The model under review builds one solid part; all positions refer to its coordinate system, in mm. A direction names the side the tool comes from. Coordinates: 2 decimals unless noted, no trailing zeros. Write each loop counter-clockwise with the first axis right and the second up, starting at its lowest first coordinate (ties: lowest second). Pieces come first, ordered by that corner, then holes. Notation, with made-up numbers: (69.5, 66) -> (74.5, 66) arc R24 cw to (74.5, 94) -> close; hole circle Ø9 at (56, 89.25). An arc over 180 degrees is marked (long way). Write each question's results on one line, items separated by ' | '.
Autodesk Inventor part; units mm, degrees
ref_plane "YZ Plane" through (0, 0, 0) normal (1, 0, 0) x (0, 1, 0)
ref_plane "XZ Plane" through (0, 0, 0) normal (0, 1, 0) x (-1, 0, 0)
ref_plane "XY Plane" through (0, 0, 0) normal (0, 0, 1) x (1, 0, 0)
sketch "Boceto1" plane through (0, 0, 0) normal (0, 0, 1) x (1, 0, 0)
  line L0 (-39, -32) -> (39, -32)
  line L1 (45.5, -25.5) -> (45.5, 25.5)
  line L2 (39, 32) -> (-39, 32)
  line L3 (-45.5, 25.5) -> (-45.5, -25.5)
  line L4 (-45.5, -32) -> (45.5, 32) construction
  line L5 (45.5, -32) -> (-45.5, 32) construction
  line L6 (-45.5, -32) -> (45.5, -32) construction
  arc A0 (-39, 32) -> (-45.5, 25.5) centre (-39, 25.5) ccw
  arc A1 (-45.5, -25.5) -> (-39, -32) centre (-39, -25.5) ccw
  arc A2 (45.5, 25.5) -> (39, 32) centre (39, 25.5) ccw
  arc A3 (39, -32) -> (45.5, -25.5) centre (39, -25.5) ccw
  line L7 (-43.5, 25.5) -> (-43.5, -25.5)
  arc A4 (-43.5, -25.5) -> (-39, -30) centre (-39, -25.5) ccw
  line L8 (-39, -30) -> (39, -30)
  arc A5 (39, -30) -> (43.5, -25.5) centre (39, -25.5) ccw
  line L9 (43.5, -25.5) -> (43.5, 25.5)
  arc A6 (43.5, 25.5) -> (39, 30) centre (39, 25.5) ccw
  line L10 (39, 30) -> (-39, 30)
  arc A7 (-39, 30) -> (-43.5, 25.5) centre (-39, 25.5) ccw
  line L11 (-42, 25.5) -> (-42, -25.5)
  arc A8 (-42, -25.5) -> (-39, -28.5) centre (-39, -25.5) ccw
  line L12 (-39, -28.5) -> (39, -28.5)
  arc A9 (39, -28.5) -> (42, -25.5) centre (39, -25.5) ccw
  line L13 (42, -25.5) -> (42, 25.5)
  arc A10 (42, 25.5) -> (39, 28.5) centre (39, 25.5) ccw
  line L14 (39, 28.5) -> (-39, 28.5)
  arc A11 (-39, 28.5) -> (-42, 25.5) centre (-39, 25.5) ccw
  circle A12 centre (-39, 24.5) radius 1.5
  circle A13 centre (-39, -24.5) radius 1.5
  circle A14 centre (19, 24.5) radius 1.5
  circle A15 centre (19, -24.5) radius 1.5
  line L15 (-42.5, 28) -> (42.5, 28) construction
  line L16 (42.5, 28) -> (42.5, -28) construction
  line L17 (42.5, -28) -> (-42.5, -28) construction
  line L18 (-42.5, -28) -> (-42.5, 28) construction
  line L19 (-42.5, 28) -> (42.5, -28) construction
  line L20 (42.5, 28) -> (-42.5, -28) construction
  point P0 (0, 0)
  dimension "d0" = 91
  dimension "d1" = 0
  dimension "d2" = 64
  dimension "d4" = 13
  dimension "d5" = 13
  dimension "d6" = 13
  dimension "d7" = 13
  dimension "d48" = 2
  dimension "d49" = 1.5
  dimension "d52" = 3
  dimension "d55" = 3
  dimension "d56" = 3
  dimension "d57" = 3
  dimension "d58" = 58
  dimension "d59" = 49
  dimension "d60" = 60
  dimension "d61" = 87
  dimension "d62" = 85
  dimension "d63" = 56
  dimension "d64" = 3.5
  dimension "d65" = 3.5
extrude "Extrusión3" add sketch "Boceto1" along normal mid plane 2.5 contours A1 L3 A0 L2 A2 L1 A3 L0 | A7 L10 A6 L9 A5 L8 A4 L7 | A11 L14 A10 L13 A9 L12 A8 L11
extrude "Extrusión4" add sketch "Boceto1" along normal mid plane 6 contours A7 L10 A6 L9 A5 L8 A4 L7
sketch "Boceto3" plane through (0, 0, 1.25) normal (0, 0, 1) x (1, 0, 0)
  arc A0 (-39, 28.5) -> (-42, 25.5) centre (-39, 25.5) ccw
  line L0 (-42, 25.5) -> (-42, -25.5)
  arc A1 (-42, -25.5) -> (-39, -28.5) centre (-39, -25.5) ccw
  line L1 (-39, -28.5) -> (39, -28.5)
  arc A2 (39, -28.5) -> (42, -25.5) centre (39, -25.5) ccw
  line L2 (42, -25.5) -> (42, 25.5)
  arc A3 (42, 25.5) -> (39, 28.5) centre (39, 25.5) ccw
  line L3 (39, 28.5) -> (-39, 28.5)
  circle A4 centre (19, -24.5) radius 1.5
  circle A5 centre (19, 24.5) radius 1.5
  circle A6 centre (-39, -24.5) radius 1.5
  circle A7 centre (-39, 24.5) radius 1.5
  circle A8 centre (-39, -24.5) radius 2.5
  circle A9 centre (-39, 24.5) radius 2.5
  circle A10 centre (19, -24.5) radius 2.5
  circle A11 centre (19, 24.5) radius 2.5
  point P0 (0, 0)
  dimension "d70" = 1
  dimension "d71" = 1
  dimension "d72" = 1
  dimension "d73" = 1
extrude "Extrusión5" add sketch "Boceto3" along normal blind 4 contours A8 | A9 | A10 | A11
properties part number "TapaIntermedia"
Q1. Clearance check with flat-ended pins moving along their axes: P1, Ø0.9, axis at y = 7, z = 2, coming from the +X side; P2, Ø0.5, axis at x = -3.5, z = -2, coming from the -Y side; P3, Ø1.9, axis at y = 8, z = -2, coming from the -X side; P4, Ø0.9, axis at y = -9.5, z = 2, coming from the -X side. State where each tip first meets the part, or that it passes through.
Solution:
P1: x = 43.5 | P2: y = -30 | P3: x = -45.5 | P4: x = -43.5
Q2. Machinability: for faces 5 (the flat face through (-1, -30, 2)), 6 (the cylindrical face through (41.14, -27.6, 2.11)), 7 (the cylindrical face through (42.217, -28.647, 2.113)), 8 (the flat face through (-43.5, 0, 2)), 9 (the flat face through (-1, -28.5, -2)), which of the approach directions +Z, -Z, +X, -X, +Y, -Y give a long, thin tool a straight path to every point of the face, cutting with its end or side? Answer none if there is none.
Solution:
face 5: +Z, +X, -X, -Y | face 6: +Z | face 7: +Z, +X, -Y | face 8: +Z, -X, +Y, -Y | face 9: -Z
Q3. For line 1 (Y direction, x = 19, z = 3.5); line 2 (Y direction, x = -19.5, z = 1.5); line 3 (X direction, y = -21, z = 2), list the stretches that pass through material, from the lowest coordinate up. Write a range as from..to.
Solution:
line 1: -27..-26, -23..-22, 22..23, 26..27 | line 2: -30..-28.5, 28.5..30 | line 3: -43.5..-42, 42..43.5
Q4. Add section C-C (y = 24.5). Count the separate pieces of the cut face and the enclosed holes in it, plus the area to 3 significant figures.
Solution:
separate pieces: 3 | enclosed holes: 0 | area: 239 mm²
Q5. Add section B-B (x = 9). Write out the cut boundary in (y, z).
Solution:
outline: (-32, -1.25) -> (-30, -1.25) -> (-30, -3) -> (-28.5, -3) -> (-28.5, -1.25) -> (28.5, -1.25) -> (28.5, -3) -> (30, -3) -> (30, -1.25) -> (32, -1.25) -> (32, 1.25) -> (30, 1.25) -> (30, 3) -> (28.5, 3) -> (28.5, 1.25) -> (-28.5, 1.25) -> (-28.5, 3) -> (-30, 3) -> (-30, 1.25) -> (-32, 1.25) -> close
Q6. Add section A-A (y = -13). Write out the cut boundary in (x, z), plus the area to 3 significant figures.
Solution:
outline: (-45.5, -1.25) -> (-43.5, -1.25) -> (-43.5, -3) -> (-42, -3) -> (-42, -1.25) -> (42, -1.25) -> (42, -3) -> (43.5, -3) -> (43.5, -1.25) -> (45.5, -1.25) -> (45.5, 1.25) -> (43.5, 1.25) -> (43.5, 3) -> (42, 3) -> (42, 1.25) -> (-42, 1.25) -> (-42, 3) -> (-43.5, 3) -> (-43.5, 1.25) -> (-45.5, 1.25) -> close | area: 238 mm²
Q7. Draft analysis for pull direction X (two halves, no side actions). For faces 1 (the flat face through (-45.5, 0, 0)), 2 (the cylindrical face through (17, 23, 3)), 3 (the flat face through (20, 23, 5.25)), 4 (the flat face through (-42, 0, -2)), state which applies: pulls with the +X half, pulls with the -X half, needs draft (parallel to the pull), parting line crosses it, or undercut.
Solution:
face 1: pulls with the -X half | face 2: undercut | face 3: needs draft | face 4: undercut
